The drawing under review shows one solid part. Ordinate dimensions are in mm from its lowest x, y, z. Coordinates: 2 decimals unless noted, no trailing zeros. Write each loop counter-clockwise with the first axis right and the second up, starting at its lowest first coordinate (ties: lowest second). Pieces come first, ordered by that corner, then holes.
1) Add section B-B, the plane x = 2. State the section outline as (y, z) points.
2) Mouldability with a two-part tool opening along Z and no side actions: class the marked faces 1, 2 and 3 as released by +Z, released by -Z, zero draft, split by the parting line, or undercut.
3) Add section A-A, the plane y = 5. State the section outline as (x, z) points.
4) Add section C-C, the plane z = 2. State the section outline as (x, y) points, then the cut area to 3 significant figures.
5) For P1, Ø1.5, axis at x = 3.5, z = 17, coming from the +Y side; P2, Ø2, axis at x = 0.5, z = 19.5, coming from the +Y side; P3, Ø3, axis at x = 5, z = 5.5, coming from the +Y side, all flat-tipped, find the tip position at first contact; note any pin that passes through.
6) For line 1 (X direction, y = 3, z = 2.5); line 2 (Y direction, x = 2.5, z = 6.25); line 3 (X direction, y = 2.25, z = 15.25), list the stretches that pass through material, from the lowest coordinate up.
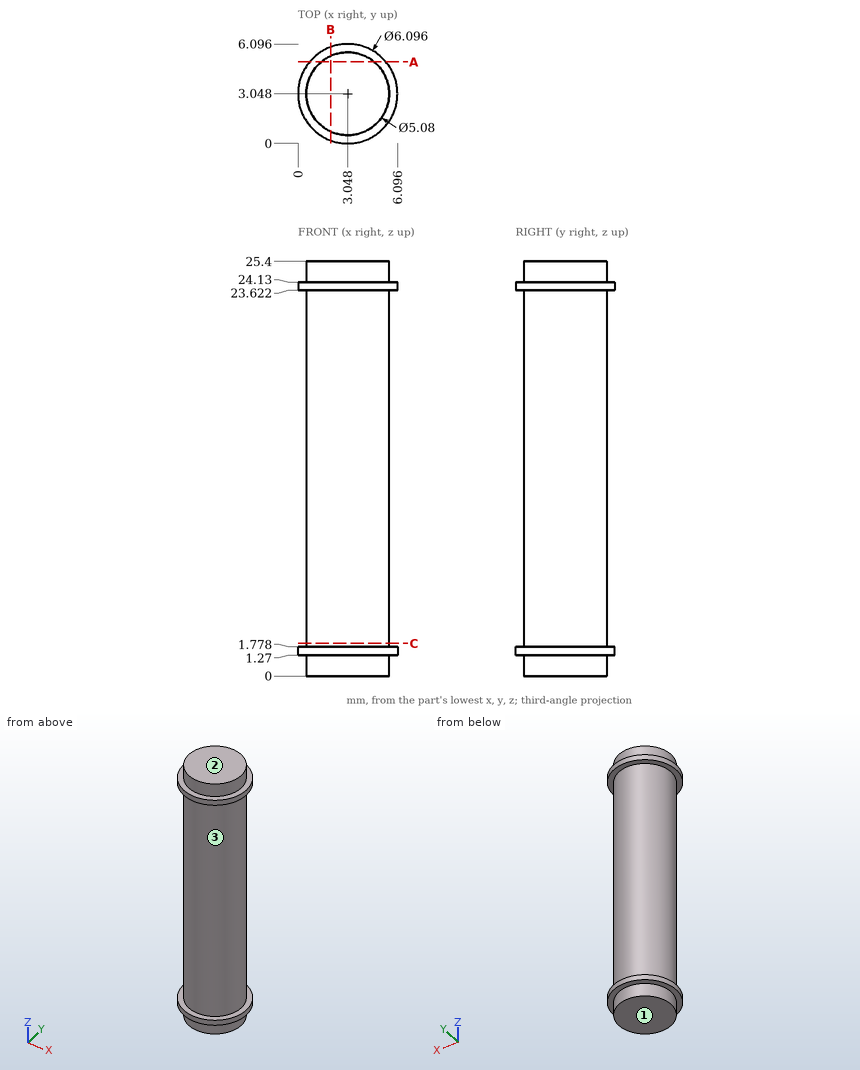
Geometry results:
1. outline: (0.19, 1.27) - (0.73, 1.27) - (0.73, 0) - (5.36, 0) - (5.36, 1.27) - (5.91, 1.27) - (5.91, 1.78) - (5.36, 1.78) - (5.36, 23.62) - (5.91, 23.62) - (5.91, 24.13) - (5.36, 24.13) - (5.36, 25.4) - (0.73, 25.4) - (0.73, 24.13) - (0.19, 24.13) - (0.19, 23.62) - (0.73, 23.62) - (0.73, 1.78) - (0.19, 1.78) - close
2. face 1: released by -Z
2. face 2: released by +Z
2. face 3: undercut
3. outline: (0.71, 1.27) - (1.42, 1.27) - (1.42, 0) - (4.67, 0) - (4.67, 1.27) - (5.39, 1.27) - (5.39, 1.78) - (4.67, 1.78) - (4.67, 23.62) - (5.39, 23.62) - (5.39, 24.13) - (4.67, 24.13) - (4.67, 25.4) - (1.42, 25.4) - (1.42, 24.13) - (0.71, 24.13) - (0.71, 23.62) - (1.42, 23.62) - (1.42, 1.78) - (0.71, 1.78) - close
4. outline: circle Ø5.08 at (3.05, 3.05)
4. area: 20.3 mm2
5. P1: stops at y = 5.59
5. P2: stops at y = 5.06
5. P3: stops at y = 5.55
6. line 1: x = 0.51 to 5.59
6. line 2: y = 0.57 to 5.53
6. line 3: x = 0.64 to 5.46
